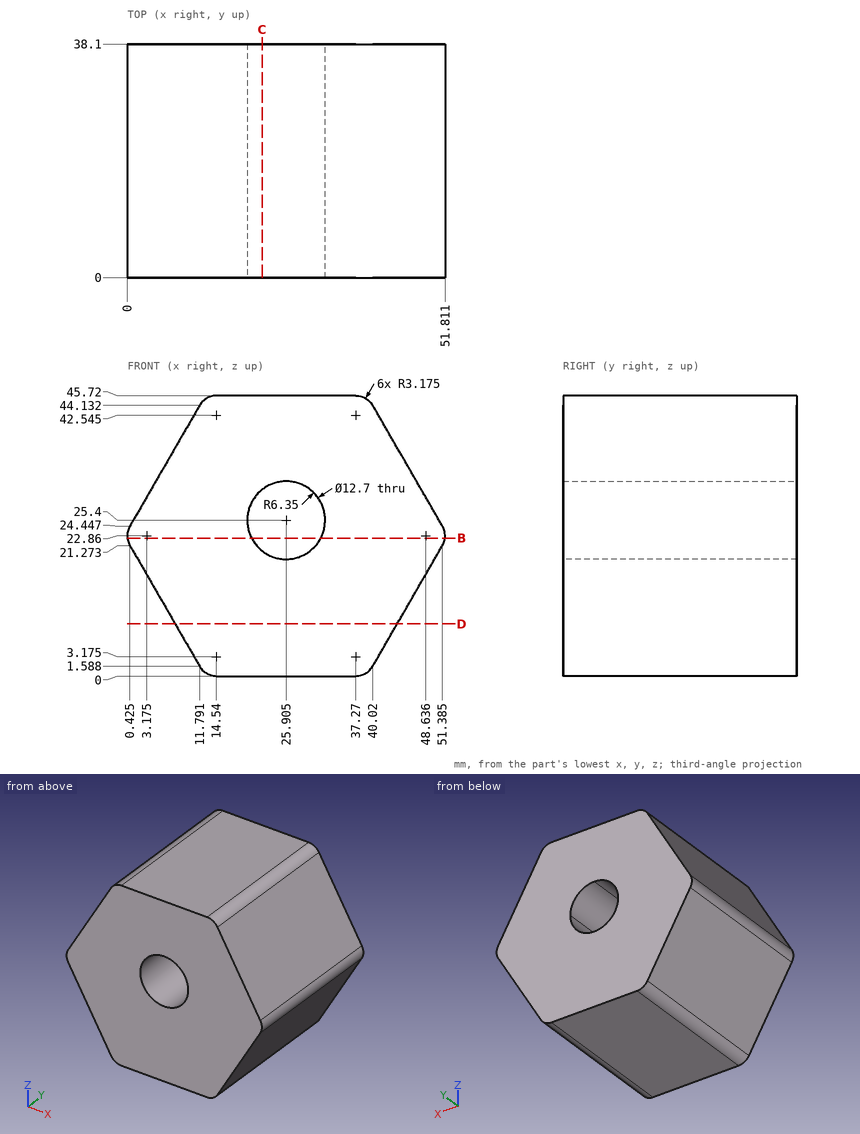
Design review of the part shown in the three views and the two pictorial views. Dimensions are in mm from the part's minimum x, y and z. Coordinates: 2 decimals unless noted, no trailing zeros. Write each loop counter-clockwise with the first axis right and the second up, starting at its lowest first coordinate (ties: lowest second). Pieces come first, ordered by that corner, then holes.
(1) Add section C-C on x = 22. Give the boundary of the cut face in (y, z), then the cut area to 3 significant figures.
(2) Add section B-B on z = 22.5. Give the boundary of the cut face in (x, y) (1 decimal).
(3) For pin 1 Ø3 at (y, z) = (32, 34) entering from -X (1 decimal); pin 2 Ø5 at (y, z) = (18, 11.5) entering from -X (1 decimal); pin 3 Ø3 at (y, z) = (5.5, 30) entering from -X (1 decimal), all flat-tipped, find the tip position at first contact; note any pin that passes through.
(4) Add section D-D on z = 8.5. Give the boundary of the cut face in (x, y).
(5) Wall thickness on probe 1 along X at (y, z) = (11, 25.4) (1 decimal); probe 2 along Z at (x, y) = (30.5, 10.5) (1 decimal); probe 3 along X at (y, z) = (20, 25) (1 decimal): over which ranges is each line inside the solid? List them lowest first.
Answer sheet:
1. outline: (0, 0) - (38.1, 0) - (38.1, 20.39) - (0, 20.39) - close; (0, 30.41) - (38.1, 30.41) - (38.1, 45.72) - (0, 45.72) - close
1. area: 1,360 mm2
2. outline: (0, 0) - (20.3, 0) - (20.3, 38.1) - (0, 38.1) - close; (31.6, 0) - (51.8, 0) - (51.8, 38.1) - (31.6, 38.1) - close
3. pin 1: stops at x = 5.1
3. pin 2: stops at x = 4.6
3. pin 3: stops at x = 2.8
4. outline: (7.8, 0) - (44.01, 0) - (44.01, 38.1) - (7.8, 38.1) - close
5. probe 1: x = 1 to 19.6, 32.3 to 50.8
5. probe 2: z = 0 to 21, 29.8 to 45.7
5. probe 3: x = 0.7 to 19.6, 32.2 to 51.1
